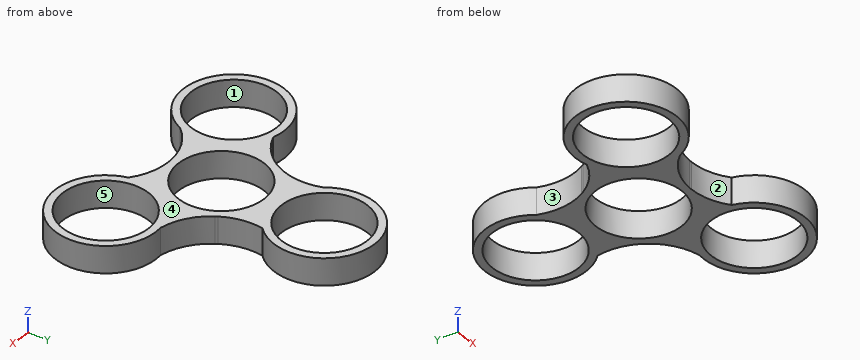
```python
from build123d import *

# Parameters (mm, degrees)
F0_R     = 11.2
F1_DEPTH = 7


with BuildPart() as f1:
    # F0 (on Top) → F1 (new body)
    with BuildSketch(Plane.XY):
        with BuildLine():
            ThreePointArc((11.102888, 7.139039), (11.269932, 6.857798), (11.442949, 6.580191))
            ThreePointArc((11.442949, 6.580191), (11.276381, 6.861722), (11.102888, 7.139039))
        make_face()
        with BuildLine():
            ThreePointArc((21.606693, -0.244218), (15.812737, 2.107464), (11.442949, 6.580191))
            ThreePointArc((11.442949, 6.580191), (11.269932, 6.857798), (11.102888, 7.139039))
            ThreePointArc((11.102888, 7.139039), (9.291098, 12.050506), (9.240533, 17.285249))
            ThreePointArc((9.240533, 17.285249), (1.027722, 39.871343), (-10.591848, 18.834054))
            ThreePointArc((-10.591848, 18.834054), (-9.731486, 12.6405), (-11.420087, 6.61979))
            ThreePointArc((-11.420087, 6.61979), (-11.573993, 6.331149), (-11.734033, 6.045864))
            ThreePointArc((-11.734033, 6.045864), (-15.081593, 2.021074), (-19.589731, -0.640088))
            ThreePointArc((-19.589731, -0.640088), (-35.043457, -19.045638), (-11.014845, -18.589836))
            ThreePointArc((-11.014845, -18.589836), (-6.081251, -14.747964), (-0.022862, -13.19998))
            ThreePointArc((-0.022862, -13.19998), (0.304061, -13.188947), (0.631145, -13.184903))
            ThreePointArc((0.631145, -13.184903), (5.790495, -14.071579), (10.349198, -16.64516))
            ThreePointArc((10.349198, -16.64516), (34.015735, -20.825705), (21.606693, -0.244218))
        make_face()
        with Locations((-23.132761, -13.355706)):
            Circle(F0_R, mode=Mode.SUBTRACT)
        with Locations((23.132761, -13.355706)):
            Circle(F0_R, mode=Mode.SUBTRACT)
        Circle(F0_R, mode=Mode.SUBTRACT)
        with Locations((0, 26.711412)):
            Circle(F0_R, mode=Mode.SUBTRACT)
        with BuildLine():
            ThreePointArc((-0.022862, -13.19998), (0.304235, -13.196494), (0.631145, -13.184903))
            ThreePointArc((0.631145, -13.184903), (0.304061, -13.188947), (-0.022862, -13.19998))
        make_face()
        with BuildLine():
            ThreePointArc((-11.734033, 6.045864), (-11.573993, 6.331149), (-11.420087, 6.61979))
            ThreePointArc((-11.420087, 6.61979), (-11.580616, 6.334772), (-11.734033, 6.045864))
        make_face()
    extrude(amount=F1_DEPTH)


solid = f1.part
```
CAD build for the part. Positions are in the model's coordinates, mm. Face numbers are marked on the shaded views. A direction names the side the tool comes from. Coordinates: 2 decimals unless noted, no trailing zeros. Loops run counter-clockwise (first coordinate to the right, second up) from the corner with the lowest first, then second, coordinate; pieces in that order, holes last. Notation, with made-up numbers: (-16.5, -4) - (31.5, -4) arc R30 cw to (31.5, 19) - close; hole circle Ø6 at (77, 22.25). An arc over 180 degrees is marked (long way). Use CSV: the item, a comma, the result in double quotes. Start each with the question number.
Q1. Drop flat-ended pins along their axis: P1, Ø4, axis at x = -12.5, y = 15.5, coming from the +Z side; P2, Ø2, axis at x = -26, z = 6, coming from the -Y side; P3, Ø4, axis at y = 9, z = 1.5, coming from the -X side. Give the stop position or say it passes through.
Q2. 3-axis set-ups, long thin cutter, end or side, ignore diameter. For the marked faces 1 and 2: which of +Z, -Z, +X, -X, +Y, -Y reach the whole face in a straight line?
Q3. Two-plate mould, pull along X, no slides. Class the marked faces 3, 4 and 5: +X half, -X half, draft (parallel to the pull), parting line (faces both ways), or undercut.
Q4. Cut at A-A, the plane y = 30. List the corners of the cut face in (x, z), then the cut area to 3 significant figures.
Q5. Cut at D-D, the plane z = 5.25. List the corners of the cut face in (x, y).
Q6. Probe probe 1 along Y at (x, z) = (0, 1.5); probe 2 along X at (y, z) = (-13, 0.75); probe 3 along X at (y, z) = (-16, 3.5). List the from-to ranges inside material, lowest first. Write a range as from..to.
Q7. Cut at C-C, the plane x = -1. List the corners of the cut face in (y, z).
Q8. Cut at B-B, the plane x = -16.5. List the corners of the cut face in (y, z).
Here are the results:
1,P1,"through"
1,P2,"y = -26.42"
1,P3,"x = -11.23"
2,face 1,"+Z, -Z"
2,face 2,"+Z, -Z, -Y"
3,face 3,"-X half"
3,face 4,"draft"
3,face 5,"undercut"
4,outline,"(-12.78, 0) - (-10.71, 0) - (-10.71, 7) - (-12.78, 7) - close; (10.71, 0) - (12.78, 0) - (12.78, 7) - (10.71, 7) - close"
4,area,"29.1 mm2"
5,outline,"(-19.59, -0.64) arc R13.2 ccw (long way) to (-11.01, -18.59) arc R15.3 cw to (-0.02, -13.2) arc R13.2 ccw to (0.63, -13.18) arc R15.3 cw to (10.35, -16.65) arc R13.2 ccw (long way) to (21.61, -0.24) arc R15.3 cw to (11.44, 6.58) arc R13.2 ccw to (11.1, 7.14) arc R15.3 cw to (9.24, 17.29) arc R13.2 ccw (long way) to (-10.59, 18.83) arc R15.3 cw to (-11.42, 6.62) arc R13.2 ccw to (-11.73, 6.05) arc R15.3 cw to start; hole circle Ø22.4 at (-23.13, -13.36); hole circle Ø22.4 at (0, 0); hole circle Ø22.4 at (0, 26.71); hole circle Ø22.4 at (23.13, -13.36)"
6,probe 1,"-13.2..-11.2, 11.2..15.51, 37.91..39.91"
6,probe 2,"-36.33..-34.33, -11.94..11.94, 34.33..36.33"
6,probe 3,"-36.07..-34.02, -12.25..-8.19, 9.5..12.25, 34.02..36.07"
7,outline,"(-13.27, 0) - (-11.16, 0) - (-11.16, 7) - (-13.27, 7) - close; (11.16, 0) - (15.56, 0) - (15.56, 7) - (11.16, 7) - close; (37.87, 0) - (39.87, 0) - (39.87, 7) - (37.87, 7) - close"
8,outline,"(-24.77, 0) - (-22.38, 0) - (-22.38, 7) - (-24.77, 7) - close; (-4.33, 0) - (0.95, 0) - (0.95, 7) - (-4.33, 7) - close"
